The listing builds one solid part. Answer for the finished solid, in the listing's coordinates (mm). A direction names the side the tool comes from. Coordinates: 2 decimals unless noted, no trailing zeros. Order: outer loops, then holes, each group sorted by start corner. A loop starts at its lowest first (then second) coordinate and runs counter-clockwise, first axis right, second up. Notation, with made-up numbers: (20.25, 50) -> (71.25, 50) arc R16 ccw to (71.25, 75) -> close; hole circle Ø4 at (66.5, -7). An arc over 180 degrees is marked (long way). Return JSON: item names as keys, results as strings.
```python
from build123d import *

# Parameters (mm, degrees)
BOSS_EXTRUDE1_DEPTH = 3
SKETCH2_R           = 1.25
CUT_EXTRUDE1_DEPTH  = 3


with BuildPart() as part:
    # Sketch1 → Boss-Extrude1 (new body)
    with BuildSketch(Plane.XY):
        Polygon((-9.553498798, 42.962261971), (-9.553498798, -1.037738029), (-17.553498798, -9.037738029), (-17.553498798, 42.962261971), align=None)
    extrude(amount=BOSS_EXTRUDE1_DEPTH)

    # Sketch2 → Cut-Extrude1 (cut)
    with BuildSketch(Plane.XY.offset(3)):
        with Locations((-13.553498798, 40.962261971)):
            Circle(SKETCH2_R)
        Polygon((-17.553498798, -9.037738029), (-17.553498798, 5.962261971), (-15.553498798, 5.962261971), (-15.553498798, -7.037738029), align=None)
    extrude(amount=-CUT_EXTRUDE1_DEPTH, mode=Mode.SUBTRACT)


solid = part.part
```
Item 1: The part is cut by section D-D on x = -16.5. Determine the outline of the cut face in (y, z), plus the area to 3 significant figures.
Answer list:
{"outline": "(5.96, 0) -> (42.96, 0) -> (42.96, 3) -> (5.96, 3) -> close", "area": "111 mm2"}
Item 2: The part is cut by section B-B on z = 2. Determine the outline of the cut face in (x, y), plus the area to 3 significant figures.
Answer list:
{"outline": "(-17.55, 5.96) -> (-15.55, 5.96) -> (-15.55, -7.04) -> (-9.55, -1.04) -> (-9.55, 42.96) -> (-17.55, 42.96) -> close; hole circle Ø2.5 at (-13.55, 40.96)", "area": "351 mm2"}
Item 3: The part is cut by section C-C on y = 0.5. Determine the outline of the cut face in (x, z), plus the area to 3 significant figures.
Answer list:
{"outline": "(-15.55, 0) -> (-9.55, 0) -> (-9.55, 3) -> (-15.55, 3) -> close", "area": "18.0 mm2"}
Item 4: The part is cut by section A-A on x = -13.25. Determine the outline of the cut face in (y, z).
Answer list:
{"outline": "(-4.73, 0) -> (39.75, 0) -> (39.75, 3) -> (-4.73, 3) -> close; (42.17, 0) -> (42.96, 0) -> (42.96, 3) -> (42.17, 3) -> close"}
Item 5: Which of the six approach directions +Z, -Z, +X, -X, +Y, -Y give full straight-line access (tool end or side, diameter ignored) to faces 4 (the flat face through (-14, 42.962, 1)), 5 (the flat face through (-15.553, 0, 2))?
Answer list:
{"face 4": "+Z, -Z, +X, -X, +Y", "face 5": "+Z, -Z, -X, -Y"}
Item 6: Flat-ended cylindrical pins translate along their axes: pin 1 (1.5 mm diameter, centred on y = -1.5, z = 1, fed in from -X); pin 2 (1 mm diameter, centred on x = -13.5, z = 1.5, fed in from -Y); pin 3 (1 mm diameter, centred on x = -14, z = 1.5, fed in from -Y); pin 4 (1.5 mm diameter, centred on x = -13.55, y = 40.96, fed in from +Z). Find the tip coordinate at first contact, or state that the pin passes through.
Answer list:
{"pin 1": "x = -15.55", "pin 2": "y = -5.48", "pin 3": "y = -5.98", "pin 4": "through"}
Item 7: Find the intervals of material crossed by probe 1 along Y at (x, z) = (-17, 1.7); probe 2 along X at (y, z) = (0, 0.9); probe 3 along Y at (x, z) = (-12.75, 1.6), in increasing order.
Answer list:
{"probe 1": "5.96 to 42.96", "probe 2": "-15.55 to -9.55", "probe 3": "-4.23 to 40, 41.92 to 42.96"}
Item 8: Determine the mould class of faces 1 (the flat face through (-12.511, -3.996, 1.479)), 2 (the flat face through (-13, 18, 3)), 3 (the flat face through (-13, 18, 0)) for opening direction Z: pulls with the +Z half, pulls with the -Z half, needs draft (parallel to the pull), parting line crosses it, or undercut.
Answer list:
{"face 1": "needs draft", "face 2": "pulls with the +Z half", "face 3": "pulls with the -Z half"}
